from build123d import *
from build123d.topology import SkipClean

# Parameters (mm, degrees)
BOSS_EXTRUDE1_DEPTH     = 2.5
SKETCH3_R               = 5.875
BOSS_EXTRUDE2_DEPTH     = 5
CUT_EXTRUDE1_DEPTH      = 55.053359054
CUT_EXTRUDE1_DEPTH_BACK = 55.053359054
SKETCH2_R               = 1.7
CUT_EXTRUDE2_DEPTH      = 55.341656443
CUT_EXTRUDE2_DEPTH_BACK = 55.341656443
SKETCH4_R               = 1.7


with BuildPart() as part:
    # Sketch1 → Boss-Extrude1 (new, symmetric)
    with BuildSketch(Plane.XY):
        with BuildLine():
            Line((-47.625, 5.875), (47.625, 5.875))
            ThreePointArc((47.625, 5.875), (53.5, 0), (47.625, -5.875))
            Line((47.625, -5.875), (-47.625, -5.875))
            ThreePointArc((-47.625, -5.875), (-53.5, 0), (-47.625, 5.875))
        make_face()
    extrude(amount=BOSS_EXTRUDE1_DEPTH, both=True)

    # Sketch3 → Boss-Extrude2 (add, symmetric)
    with SkipClean():  # the faces are left unmerged after this step: merging them gives an invalid solid
        with BuildSketch(Plane.XY):
            with Locations((-47.625, 0)):
                Circle(SKETCH3_R)
            with Locations((47.625, 0)):
                Circle(SKETCH3_R)
        extrude(amount=BOSS_EXTRUDE2_DEPTH, both=True)
    add(part.part.scale(1), mode=Mode.REPLACE)  # the faces are merged on a copy

    # Sketch2 → Cut-Extrude1 (cut, two sides: drawn at the far end of the back side and taken through both)
    with BuildSketch(Plane.XY.offset(-CUT_EXTRUDE1_DEPTH_BACK)):
        with Locations((-47.625, 0)):
            Circle(SKETCH2_R)
        with Locations((47.625, 0)):
            Circle(SKETCH2_R)
    extrude(amount=CUT_EXTRUDE1_DEPTH + CUT_EXTRUDE1_DEPTH_BACK, mode=Mode.SUBTRACT)

    # Sketch4 → Cut-Extrude2 (cut, two sides: drawn at the far end of the back side and taken through both)
    with BuildSketch(Plane.XY.offset(2.5).offset(-CUT_EXTRUDE2_DEPTH_BACK)):
        with Locations((33.425, 0)):
            Circle(SKETCH4_R)
        with Locations((27.425, 0)):
            Circle(SKETCH4_R)
        with Locations((39.425, 0)):
            Circle(SKETCH4_R)
    extrude(amount=CUT_EXTRUDE2_DEPTH + CUT_EXTRUDE2_DEPTH_BACK, mode=Mode.SUBTRACT)


solid = part.part
Source: CAD feature listing. Evaluate the final solid. Frame: model axes, mm. Round coordinates to 2 decimals unless told otherwise and drop trailing zeros. Write each loop counter-clockwise with the first axis right and the second up, starting at its lowest first coordinate (ties: lowest second). Pieces come first, ordered by that corner, then holes. Notation, with made-up numbers: M -15,40.5 L -6,40.5 A19 ccw -6,44.5 Z; hole C 50,30.25 d11. An arc over 180 degrees is marked long. One line per item, written item: value. Start each with the question number.
Item 1: Section query C-C (x = -7). Return the cut outline in (y, z) (3 decimals), plus the area to 4 significant figures.
Item 2: Section query B-B (z = 1.25). Return the cut outline in (x, y) (3 decimals), plus the area to 3 significant figures.
Item 3: Section query D-D (y = -4.5). Return the cut outline in (x, z), plus the area to 3 significant figures.
Item 4: Pin query (flat end, axial travel): pin 1 (1.5 mm diameter, centred on y = -2.5, z = 0, fed in from +X); pin 2 (4 mm diameter, centred on x = 39.425, y = 0, fed in from -Z); pin 3 (5 mm diameter, centred on y = 4.5, z = 3, fed in from +X). Return the tip coordinate at first contact, or that it passes through.
Item 5: Ray query, L1, parallel to X at y = 0, z = -0.25 (3 decimals); L2, parallel to Z at x = 36.5, y = 1.75; L3, parallel to X at y = 1, z = 0.25. Return the intervals inside material, ascending. Write a range as from..to.
Item 6: Section query A-A (y = 0). State how many separate pieces and enclosed holes the cut face has, plus the area to 4 significant figures.
Result set:
1. outline: M -5.875,-2.5 L 5.875,-2.5 L 5.875,2.5 L -5.875,2.5 Z
1. area: 58.75 mm²
2. outline: M -47.625,-5.875 L 47.625,-5.875 A5.875 ccw 47.625,5.875 L -47.625,5.875 A5.875 ccw Z; hole C -47.625,0 d3.4; hole C 27.425,0 d3.4; hole C 33.425,0 d3.4; hole C 39.425,0 d3.4; hole C 47.625,0 d3.4
2. area: 1,180 mm²
3. outline: M -51.4,-5 L -43.85,-5 L -43.85,-2.5 L 43.85,-2.5 L 43.85,-5 L 51.4,-5 L 51.4,5 L 43.85,5 L 43.85,2.5 L -43.85,2.5 L -43.85,5 L -51.4,5 Z
3. area: 590 mm²
4. pin 1: stops at x = 53.23
4. pin 2: stops at z = -2.5
4. pin 3: stops at x = 53.15
5. L1: x = -53.5..-49.325, -45.925..25.725, 29.125..31.725, 35.125..37.725, 41.125..45.925, 49.325..53.5
5. L2: z = -2.5..2.5
5. L3: x = -53.41..-49, -46.25..26.05, 28.8..32.05, 34.8..38.05, 40.8..46.25, 49..53.41
6. separate pieces: 6
6. enclosed holes: 0
6. area: 533.5 mm²
